from build123d import *

# Parameters (mm, degrees)
ESQUISSE1_R                  = 13.875
BOSS_EXTRU_1_DEPTH           = 5
ESQUISSE2_R                  = 2.625
ENL_V_MAT_EXTRU_1_DEPTH      = 2
ESQUISSE3_R                  = 3.875
BOSS_EXTRU_2_DEPTH           = 50
ESQUISSE4_R                  = 5.875
BOSS_EXTRU_3_DEPTH           = 17
ENL_V_MAT_EXTRU_2_DEPTH      = 59.395472855
ENL_V_MAT_EXTRU_2_DEPTH_BACK = 59.395472855
ESQUISSE5_R                  = 1.75
ENL_V_MAT_EXTRU_3_DEPTH      = 3


with BuildPart() as part:
    # Esquisse1 → Boss.-Extru.1 (new body)
    with BuildSketch(Plane.XY):
        Circle(ESQUISSE1_R)
    extrude(amount=BOSS_EXTRU_1_DEPTH)

    # Esquisse2 → Enlèv. mat.-Extru.1 (cut)
    with BuildSketch(Plane(origin=(0, 0, 0), x_dir=(-1, 0, 0), z_dir=(0, 0, -1))):
        Circle(ESQUISSE2_R)
    extrude(amount=-ENL_V_MAT_EXTRU_1_DEPTH, mode=Mode.SUBTRACT)

    # Esquisse3 → Boss.-Extru.2 (add)
    with BuildSketch(Plane.XY.offset(5)):
        Circle(ESQUISSE3_R)
    extrude(amount=BOSS_EXTRU_2_DEPTH)

    # Esquisse4 → Boss.-Extru.3 (add)
    with BuildSketch(Plane.XY.offset(5)):
        Circle(ESQUISSE4_R)
    extrude(amount=BOSS_EXTRU_3_DEPTH)

    # Esquisse5 → Enlèv. mat.-Extru.2 (cut, two sides: drawn at the far end of the back side and taken through both)
    with BuildSketch(Plane(origin=(0, 0, 0), x_dir=(-1, 0, 0), z_dir=(0, 0, -1)).offset(-ENL_V_MAT_EXTRU_2_DEPTH_BACK)):
        with Locations((9.987504748, 0.499748848)):
            Circle(ESQUISSE5_R)
        with Locations((-4.560957176, -8.899307256)):
            Circle(ESQUISSE5_R)
        with Locations((-5.426547571, 8.399558408)):
            Circle(ESQUISSE5_R)
    extrude(amount=ENL_V_MAT_EXTRU_2_DEPTH + ENL_V_MAT_EXTRU_2_DEPTH_BACK, mode=Mode.SUBTRACT)

    # Esquisse6 → Enlèv. mat.-Extru.3 (cut)
    with BuildSketch(Plane(origin=(0, 0, 0), x_dir=(-1, 0, 0), z_dir=(0, 0, -1))):
        with BuildLine():
            Line((9.787605209, 4.494750747), (14.846993763, 4.747909435))
            ThreePointArc((14.846993763, 4.747909435), (19.041895201, 0.952807075), (15.246792841, -3.242094364))
            Line((15.246792841, -3.242094364), (10.187404287, -3.495253052))
            ThreePointArc((10.187404287, -3.495253052), (5.992502849, 0.299849309), (9.787605209, 4.494750747))
        make_face()
        with BuildLine():
            Line((-1.001234274, -10.723690126), (-4.262940688, -17.087908521))
            ThreePointArc((-4.262940688, -17.087908521), (-9.647046461, -18.823248552), (-11.382386493, -13.43914278))
            Line((-11.382386493, -13.43914278), (-8.120680079, -7.074924385))
            ThreePointArc((-8.120680079, -7.074924385), (-2.736574306, -5.339584354), (-1.001234274, -10.723690126))
        make_face()
        with BuildLine():
            Line((-8.786370935, 6.22893938), (-13.208101845, 13.073178107))
            ThreePointArc((-13.208101845, 13.073178107), (-12.01889751, 18.603620499), (-6.488455118, 17.414416164))
            Line((-6.488455118, 17.414416164), (-2.066724208, 10.570177437))
            ThreePointArc((-2.066724208, 10.570177437), (-3.255928543, 5.039735045), (-8.786370935, 6.22893938))
        make_face()
    extrude(amount=-ENL_V_MAT_EXTRU_3_DEPTH, mode=Mode.SUBTRACT)


solid = part.part
Can you work these out from the model? Positions are in its coordinate system, mm. A direction names the side the tool comes from. Round coordinates to 2 decimals unless told otherwise and drop trailing zeros. Write each loop counter-clockwise with the first axis right and the second up, starting at its lowest first coordinate (ties: lowest second). Pieces come first, ordered by that corner, then holes. Notation, with made-up numbers: M 83.5,66 L 117.5,66 A31 ccw 117.5,97 Z; hole C 27,3 d11. An arc over 180 degrees is marked long. Use a Markdown table: item, result.
Item 1: For pin 1 Ø2 at (x, y) = (-6.5, 5.5) entering from +Z; pin 2 Ø4 at (x, y) = (6.5, -3) entering from -Z; pin 3 Ø8 at (x, y) = (-1.5, 8) entering from +Z; pin 4 Ø4 at (x, z) = (5.5, 43) entering from -Y, each with a flat end and sliding along its axis, tell me the tip position at first contact or that it passes through.
Found:
| item | result |
|---|---|
| pin 1 | stops at z = 5 |
| pin 2 | stops at z = 0 |
| pin 3 | stops at z = 22 |
| pin 4 | stops at y = -1.66 |
Item 2: We'd pull the mould along Y, two halves only. Please class faces 5 (the face through (-2.5, 0.8, 1)), 6 (the face through (7, 10, 3)), 7 (the face through (8.88, -8.56, 1.48)), 8 (the face through (9.665, 7.59, 1.479)): released by +Y, released by -Y, zero draft, split by the parting line, or undercut.
Found:
| item | result |
|---|---|
| face 5 | undercut |
| face 6 | undercut |
| face 7 | released by -Y |
| face 8 | released by +Y |
Item 3: I want a section at A-A (x = 0). List the corners of the cut face in (y, z) for me (3 decimals).
Found:
| item | result |
|---|---|
| outline | M -13.875,0 L -2.625,0 L -2.625,2 L 2.625,2 L 2.625,0 L 13.875,0 L 13.875,5 L 5.875,5 L 5.875,22 L 3.875,22 L 3.875,55 L -3.875,55 L -3.875,22 L -5.875,22 L -5.875,5 L -13.875,5 Z |
Item 4: I want a section at B-B (y = 1.25). List the corners of the cut face in (x, z) for me, and give its area (3 significant figures).
Found:
| item | result |
|---|---|
| outline | M -13.82,3 L -11.57,3 L -11.57,5 L -13.82,5 Z; M -8.41,3 L -6.06,3 L -6.06,0 L -2.31,0 L -2.31,2 L 2.31,2 L 2.31,0 L 13.82,0 L 13.82,5 L 5.74,5 L 5.74,22 L 3.67,22 L 3.67,55 L -3.67,55 L -3.67,22 L -5.74,22 L -5.74,5 L -8.41,5 Z |
| area | 537 mm2 |
Item 5: If I drill on line 1 along Z through (x, y) = (0.75, -10); line 2 along Z through (x, y) = (11.25, -2.5); line 3 along X through (y, z) = (-0.25, 50), over which ranges is the centre line in solid material (lowest first)? Write a range as [from, to].
Found:
| item | result |
|---|---|
| line 1 | z = [3, 5] |
| line 2 | z = [0, 5] |
| line 3 | x = [-3.87, 3.87] |
Item 6: Which directions (+Z, -Z, +X, -X, +Y, -Y) give clear straight access to the entire face, cutting with the end or side of a thin tool? Please do faces 1 (the face through (6, -10.2, 3)), 2 (the face through (1, -4, 22)), 3 (the face through (2.97, 11.97, 1.48)), 4 (the face through (-11.406, 4.576, 1.479)).
Found:
| item | result |
|---|---|
| face 1 | -Z |
| face 2 | +Z |
| face 3 | -Z, +X |
| face 4 | -Z, -X |
Item 7: I want a section at C-C (z = 36.5). List the corners of the cut face in (x, y) for me (3 decimals), and give its area (3 significant figures).
Found:
| item | result |
|---|---|
| outline | C 0,0 d7.75 |
| area | 47.2 mm2 |
Item 8: I want a section at D-D (z = 6.5). List the corners of the cut face in (x, y) for me (3 decimals).
Found:
| item | result |
|---|---|
| outline | C 0,0 d11.75 |
